For this review, take the finished solid that the model builds, in its own axes (mm). Face numbers are marked on the shaded views. A direction names the side the tool comes from. Round coordinates to 2 decimals unless told otherwise and drop trailing zeros. Loops run counter-clockwise (first coordinate to the right, second up) from the corner with the lowest first, then second, coordinate; pieces in that order, holes last. Notation, with made-up numbers: (82, -24.5) -> (107, -24.5) arc R22 ccw to (107, -4.5) -> close; hole circle Ø8 at (79.5, -34). An arc over 180 degrees is marked (long way). Write each question's results on one line, items separated by ' | '.
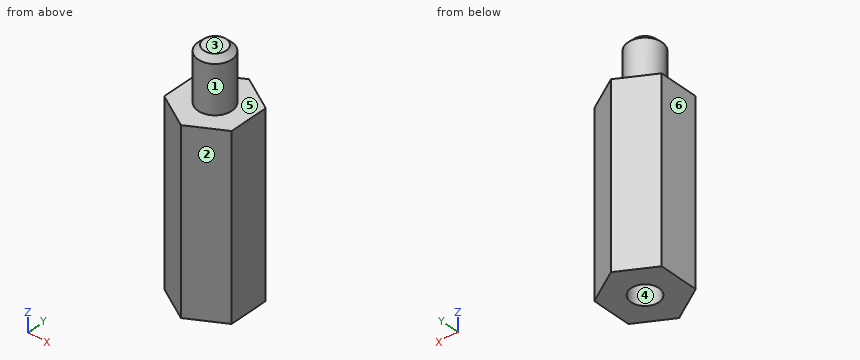
Autodesk Inventor part; units mm, degrees
ref_plane "YZ Plane" through (0, 0, 0) normal (1, 0, 0) x (0, 1, 0)
ref_plane "XZ Plane" through (0, 0, 0) normal (0, 1, 0) x (-1, 0, 0)
ref_plane "XY Plane" through (0, 0, 0) normal (0, 0, 1) x (1, 0, 0)
sketch "Sketch1" plane through (0, 0, 0) normal (0, 0, 1) x (1, 0, 0)
  line L0 (0, 3.4641) -> (3, 1.7321)
  line L1 (3, 1.7321) -> (3, -1.7321)
  line L2 (3, -1.7321) -> (0, -3.4641)
  line L3 (0, -3.4641) -> (-3, -1.7321)
  line L4 (-3, -1.7321) -> (-3, 1.7321)
  line L5 (-3, 1.7321) -> (0, 3.4641)
  point P0 (0, 0)
  point P1 (0, 0)
  dimension "d0" = 6
extrude "Extrusion1" add sketch "Sketch1" along normal blind 16
sketch "Sketch2" plane through (0, 0, 16) normal (0, 0, 1) x (1, 0, 0)
  circle A0 centre (0, 0) radius 1.5
  dimension "d3" = 3
extrude "Extrusion2" add sketch "Sketch2" along normal blind 4.76
thread "Thread1"
sketch "Sketch3" plane through (0, 0, 0) normal (0, 0, -1) x (-1, 0, 0)
  point P0 (0, 0)
hole "Hole1" at (0, 0, 0) direction (0, 0, 1) diameter 2.459 depth 6.4 tip angle 118
chamfer "Chamfer1" distance 0.5 angle 45 1 edges at (-1.5, 0, 20.76)
properties part number "3mm-standoff-16-long"
1. Consider section A-A (z = 7.75). State the section outline as (x, y) points.
Values found:
outline: (-3, -1.73) -> (0, -3.46) -> (3, -1.73) -> (3, 1.73) -> (0, 3.46) -> (-3, 1.73) -> close
2. Tool access review of the marked faces 5 and 6: name each direction out of +Z, -Z, +X, -X, +Y, -Y from which nothing blocks a thin tool from reaching the whole face with its end or side.
Values found:
face 5: +Z | face 6: +Z, -Z, -X, +Y, -Y
3. Draft analysis for pull direction Y (two halves, no side actions). For the marked faces 1, 2, 3 and 4, state which applies: released by +Y, released by -Y, zero draft, split by the parting line, or undercut.
Values found:
face 1: split by the parting line | face 2: released by -Y | face 3: zero draft | face 4: undercut
4. To check wall thickness, follow probe 1 along X at (y, z) = (0, 2); probe 2 along Z at (x, y) = (-1.7, 1.5); probe 3 along Y at (x, z) = (-0.55, 3.5). State the ranges of each line that lie inside material, in increasing order.
Values found:
probe 1: x = -3 to -1.23, 1.23 to 3 | probe 2: z = 0 to 16 | probe 3: y = -3.15 to -1.1, 1.1 to 3.15
5. For pin 1 (1.5 mm diameter, centred on x = 1, y = 1.5, fed in from +Z); pin 2 (1.5 mm diameter, centred on x = 0, y = 0, fed in from -Z), all flat-tipped, find the tip position at first contact; note any pin that passes through.
Values found:
pin 1: stops at z = 20.71 | pin 2: stops at z = 6.69
